Work out the finished part from the listing and answer in its coordinate system (mm). A direction names the side the tool comes from. Round coordinates to 2 decimals unless told otherwise and drop trailing zeros. Order: outer loops, then holes, each group sorted by start corner. A loop starts at its lowest first (then second) coordinate and runs counter-clockwise, first axis right, second up. Notation, with made-up numbers: M 26.25,-40 L 73.25,-40 A19 cw 73.25,-26 Z; hole C 6,9.25 d8. An arc over 180 degrees is marked long. Return JSON: item names as keys, results as strings.
from build123d import *

# Parameters (mm, degrees)
SKETCH1_W           = 74.870479659
SKETCH1_H           = 36.98000569
BOSS_EXTRUDE1_DEPTH = 12
SKETCH3_R           = 1.651
BOSS_EXTRUDE2_DEPTH = 18
SKETCH4_W           = 15
SKETCH4_H           = 15
BOSS_EXTRUDE3_DEPTH = 18
SKETCH5_R           = 4.075
SKETCH5_R_2         = 4.25
CUT_EXTRUDE1_DEPTH  = 12
BOSS_EXTRUDE4_DEPTH = 36.980006


with BuildPart() as part:
    # Sketch1 → Boss-Extrude1 (new body)
    with BuildSketch(Plane.ZY.offset(-34.568450848)):
        with Locations((-283.368991002, -85.966002845)):
            Rectangle(SKETCH1_W, SKETCH1_H)
    extrude(amount=BOSS_EXTRUDE1_DEPTH)

    # Sketch3 → Boss-Extrude2 (add)
    with BuildSketch(Plane(origin=(34.568450848, 0, 0), x_dir=(0, 0, -1), z_dir=(1, 0, 0))):
        with Locations((271.241893694, -74.826)):
            Circle(SKETCH3_R)
        with Locations((271.241893694, -90.126)):
            Circle(SKETCH3_R)
        with Locations((294.241893694, -74.826)):
            Circle(SKETCH3_R)
        with Locations((294.241893694, -90.126)):
            Circle(SKETCH3_R)
    extrude(amount=BOSS_EXTRUDE2_DEPTH)

    # Sketch4 → Boss-Extrude3 (add)
    with BuildSketch(Plane(origin=(34.568450848, 0, 0), x_dir=(0, 0, -1), z_dir=(1, 0, 0))):
        with Locations((253.433751172, -96.95600569)):
            Rectangle(SKETCH4_W, SKETCH4_H)
        with Locations((313.304230831, -96.95600569)):
            Rectangle(SKETCH4_W, SKETCH4_H)
    extrude(amount=BOSS_EXTRUDE3_DEPTH)

    # Sketch5 → Cut-Extrude1 (cut)
    with BuildSketch(Plane.XZ.offset(104.45600569)):
        with Locations((45.518450848, -252.717)):
            Circle(SKETCH5_R)
        with Locations((45.518450848, -311.899)):
            Circle(SKETCH5_R_2)
    extrude(amount=-CUT_EXTRUDE1_DEPTH, mode=Mode.SUBTRACT)

    # Sketch7 → Boss-Extrude4 (add)
    with BuildSketch(Plane(origin=(0, -67.476, 0), x_dir=(1, 0, 0), z_dir=(0, 1, 0))):
        with BuildLine():
            Line((8.49017791, 282.708508335), (8.49017791, 281.891491665))
            ThreePointArc((8.49017791, 281.891491665), (8.198108508, 280.0547791), (7.513571814, 278.325551788))
            ThreePointArc((7.513571814, 278.325551788), (7.368274769, 277.471769831), (7.758499153, 276.698607628))
            Line((7.758499153, 276.698607628), (11.301449673, 273.155657108))
            ThreePointArc((11.301449673, 273.155657108), (11.750776011, 272.855426847), (12.280792565, 272.75))
            Line((12.280792565, 272.75), (16.2, 272.75))
            Line((16.2, 272.75), (16.2, 276.923))
            ThreePointArc((16.2, 276.923), (16.456867353, 277.543132647), (17.077, 277.8))
            Line((17.077, 277.8), (20.8615, 277.8))
            Line((20.8615, 277.8), (22.568450848, 277.8))
            Line((22.568450848, 277.8), (22.568450848, 286.8))
            Line((22.568450848, 286.8), (20.8615, 286.8))
            Line((20.8615, 286.8), (17.077, 286.8))
            ThreePointArc((17.077, 286.8), (16.456867353, 287.056867353), (16.2, 287.677))
            Line((16.2, 287.677), (16.2, 291.85))
            Line((16.2, 291.85), (12.280792565, 291.85))
            ThreePointArc((12.280792565, 291.85), (11.750776011, 291.744573153), (11.301449673, 291.444342892))
            Line((11.301449673, 291.444342892), (7.758499153, 287.901392372))
            ThreePointArc((7.758499153, 287.901392372), (7.368274769, 287.128230169), (7.513571814, 286.274448212))
            ThreePointArc((7.513571814, 286.274448212), (8.198108508, 284.5452209), (8.49017791, 282.708508335))
        make_face()
    extrude(amount=-BOSS_EXTRUDE4_DEPTH)


solid = part.part
Item 1: Find section B-B (z = -274). Determine the outline of the cut face in (x, y).
Output:
{"outline": "M 10.46,-104.46 L 16.2,-104.46 L 16.2,-67.48 L 10.46,-67.48 Z; M 22.57,-104.46 L 34.57,-104.46 L 34.57,-67.48 L 22.57,-67.48 Z"}
Item 2: Find section D-D (z = -283.5). Determine the outline of the cut face in (x, y), plus the area to 3 significant figures.
Output:
{"outline": "M 8.41,-104.46 L 34.57,-104.46 L 34.57,-67.48 L 8.41,-67.48 Z", "area": "967 mm^2"}
Item 3: Consider line 1 along Z through (x, y) = (40.5, -95); line 2 along X through (y, z) = (-84, -262.5); line 3 along Y through (x, z) = (49.5, -316). Determine where each line is inside the solid, lowest interval first. Write a range as [from, to].
Output:
{"line 1": "z = [-320.8, -305.8], [-260.93, -245.93]", "line 2": "x = [22.57, 34.57]", "line 3": "y = [-104.46, -89.46]"}
Item 4: Each of these flat-tipped pins is pushed along its axis until it touches: pin 1 (2 mm diameter, centred on x = 14.5, y = -87, fed in from +Z); pin 2 (2 mm diameter, centred on y = -93.5, z = -274.5, fed in from +X); pin 3 (4.5 mm diameter, centred on x = 19.5, y = -90, fed in from -Z); pin 4 (13.5 mm diameter, centred on x = 45.52, z = -311.9, fed in from -Y). Where does it stop, or does it pass through?
Output:
{"pin 1": "stops at z = -272.75", "pin 2": "stops at x = 34.57", "pin 3": "stops at z = -286.8", "pin 4": "stops at y = -104.46"}
Item 5: Which of the six approach directions +Z, -Z, +X, -X, +Y, -Y give full straight-line access (tool end or side, diameter ignored) to faces 4 (the flat face through (14, -86, -272.75)), 5 (the cylindrical face through (47.4, -98.54, -256.33)), 6 (the flat face through (16.2, -86, -290)), 7 (the flat face through (43, -89.456, -253)), 8 (the flat face through (43, -89.456, -313))?
Output:
{"face 4": "+Z, -X, +Y, -Y", "face 5": "-Y", "face 6": "-Z, +Y, -Y", "face 7": "+Z, +X, +Y", "face 8": "-Z, +X, +Y"}
Item 6: Find section A-A (x = 47.5). Determine the outline of the cut face in (y, z).
Output:
{"outline": "M -104.46,-320.8 L -89.46,-320.8 L -89.46,-305.8 L -104.46,-305.8 L -104.46,-308.14 L -92.46,-308.14 L -92.46,-315.66 L -104.46,-315.66 Z; M -104.46,-260.93 L -89.46,-260.93 L -89.46,-245.93 L -104.46,-245.93 L -104.46,-249.16 L -92.46,-249.16 L -92.46,-256.28 L -104.46,-256.28 Z; C -90.13,-294.24 d3.3; C -90.13,-271.24 d3.3; C -74.83,-294.24 d3.3; C -74.83,-271.24 d3.3"}
Item 7: The mould has two halves that part along X. Classify faces 1 (the cylindrical face through (7.366, -85.707, -277.484)), 2 (the cylindrical face through (43.44, -91.13, -269.93)), 3 (the flat face through (20, -86, -286.8)): pulls with the +X half, pulls with the -X half, needs draft (parallel to the pull), parting line crosses it, or undercut.
Output:
{"face 1": "pulls with the -X half", "face 2": "needs draft", "face 3": "undercut"}
